from build123d import *

# Parameters (mm, degrees)
SKETCH3_R            = 27.94
BOSS_EXTRUDE2_DEPTH  = 122.46
SKETCH5_R            = 3.175
CUT_EXTRUDE1_DEPTH   = 129.676877488
SKETCH4_W            = 14
SKETCH4_H            = 6
SHELL1_START         = 3
SHELL1_OUTLINE_R     = 10.94
SHELL1_OUTLINE_R_2   = 6.175
SHELL1_DEPTH         = 116.46
SHELL1_2_OUTLINE_R   = 24.94
SHELL1_2_OUTLINE_R_2 = 10.94
SHELL1_2_DEPTH       = 10.72
SHELL1_START_2       = 109.72
SHELL1_3_OUTLINE_R   = 24.94
SHELL1_3_OUTLINE_R_2 = 10.94
SHELL1_3_DEPTH       = 9.74
SHELL1_START_3       = 25.72
SHELL1_4_OUTLINE_R   = 24.94
SHELL1_4_OUTLINE_R_2 = 10.94
SHELL1_4_DEPTH       = 9
SHELL1_START_4       = 46.72
SHELL1_5_OUTLINE_R   = 24.94
SHELL1_5_OUTLINE_R_2 = 10.94
SHELL1_5_DEPTH       = 9
SHELL1_START_5       = 67.72
SHELL1_6_OUTLINE_R   = 24.94
SHELL1_6_OUTLINE_R_2 = 10.94
SHELL1_6_DEPTH       = 9
SHELL1_START_6       = 88.72
SHELL1_7_OUTLINE_R   = 24.94
SHELL1_7_OUTLINE_R_2 = 10.94
SHELL1_7_DEPTH       = 9
BOSS_EXTRUDE3_REACH  = 130.677
SKETCH13_W           = 16.483162312
SKETCH13_H           = 6
CUT_EXTRUDE3_DEPTH   = 123
BOSS_EXTRUDE5_START  = -122.46
BOSS_EXTRUDE5_DEPTH  = 122.46


# Read off the part's stored shape, not the designer's step: Shell1
with BuildPart() as part:
    # Sketch3 → Boss-Extrude2 (new body)
    with BuildSketch(Plane.XY):
        Circle(SKETCH3_R)
    extrude(amount=BOSS_EXTRUDE2_DEPTH)

    # Sketch5 → Cut-Extrude1 (cut, through all)
    with BuildSketch(Plane.XY.offset(122.46)):
        Circle(SKETCH5_R)
    extrude(amount=-CUT_EXTRUDE1_DEPTH, mode=Mode.SUBTRACT)

    # Sketch4 → Cut-Revolve1 (revolve, cut)
    with BuildSketch(Plane(origin=(0, 0, 0), x_dir=(1, 0, 0), z_dir=(0, 1, 0)), mode=Mode.PRIVATE) as cut_revolve1_sk:
        with Locations((-20.94, -103.72)):
            Rectangle(SKETCH4_W, SKETCH4_H)
        with Locations((-20.94, -82.72)):
            Rectangle(SKETCH4_W, SKETCH4_H)
        with Locations((-20.94, -61.72)):
            Rectangle(SKETCH4_W, SKETCH4_H)
        with Locations((-20.94, -40.72)):
            Rectangle(SKETCH4_W, SKETCH4_H)
        with Locations((-20.94, -19.72)):
            Rectangle(SKETCH4_W, SKETCH4_H)
    revolve(cut_revolve1_sk.sketch.rotate(Axis((0, 0, 122.46), (0, 0, -1)), 180), axis=Axis((0, 0, 122.46), (0, 0, -1)), mode=Mode.SUBTRACT)

    # Shell1 outline → Shell1 (cut)
    with BuildSketch(Plane.XY.offset(SHELL1_START)):
        Circle(SHELL1_OUTLINE_R)
        Circle(SHELL1_OUTLINE_R_2, mode=Mode.SUBTRACT)
    extrude(amount=SHELL1_DEPTH, mode=Mode.SUBTRACT)

    # Shell1 2 outline → Shell1 2 (cut)
    with BuildSketch(Plane.XY.offset(SHELL1_START)):
        Circle(SHELL1_2_OUTLINE_R)
        Circle(SHELL1_2_OUTLINE_R_2, mode=Mode.SUBTRACT)
    extrude(amount=SHELL1_2_DEPTH, mode=Mode.SUBTRACT)

    # Shell1 3 outline → Shell1 3 (cut)
    with BuildSketch(Plane.XY.offset(SHELL1_START_2)):
        Circle(SHELL1_3_OUTLINE_R)
        Circle(SHELL1_3_OUTLINE_R_2, mode=Mode.SUBTRACT)
    extrude(amount=SHELL1_3_DEPTH, mode=Mode.SUBTRACT)

    # Shell1 4 outline → Shell1 4 (cut)
    with BuildSketch(Plane.XY.offset(SHELL1_START_3)):
        Circle(SHELL1_4_OUTLINE_R)
        Circle(SHELL1_4_OUTLINE_R_2, mode=Mode.SUBTRACT)
    extrude(amount=SHELL1_4_DEPTH, mode=Mode.SUBTRACT)

    # Shell1 5 outline → Shell1 5 (cut)
    with BuildSketch(Plane.XY.offset(SHELL1_START_4)):
        Circle(SHELL1_5_OUTLINE_R)
        Circle(SHELL1_5_OUTLINE_R_2, mode=Mode.SUBTRACT)
    extrude(amount=SHELL1_5_DEPTH, mode=Mode.SUBTRACT)

    # Shell1 6 outline → Shell1 6 (cut)
    with BuildSketch(Plane.XY.offset(SHELL1_START_5)):
        Circle(SHELL1_6_OUTLINE_R)
        Circle(SHELL1_6_OUTLINE_R_2, mode=Mode.SUBTRACT)
    extrude(amount=SHELL1_6_DEPTH, mode=Mode.SUBTRACT)

    # Shell1 7 outline → Shell1 7 (cut)
    with BuildSketch(Plane.XY.offset(SHELL1_START_6)):
        Circle(SHELL1_7_OUTLINE_R)
        Circle(SHELL1_7_OUTLINE_R_2, mode=Mode.SUBTRACT)
    extrude(amount=SHELL1_7_DEPTH, mode=Mode.SUBTRACT)

    # Boss-Extrude3: up to this face of the body (flat: up to its plane)
    boss_extrude3_end = Plane(part.part.faces().sort_by_distance((-27.149737461, 0, 122.46))[0])
    # Sketch10 → Boss-Extrude3 (add, up to the picked face)
    with BuildSketch(Plane(origin=(0, 0, 0), x_dir=(-1, 0, 0), z_dir=(0, 0, -1)), mode=Mode.PRIVATE) as boss_extrude3_sk1:
        with BuildLine():
            Line((-1, 27.922098775), (-1, 3.01340754))
            ThreePointArc((-1, 3.01340754), (0, 3.175), (1, 3.01340754))
            Line((1, 3.01340754), (1, 27.922098775))
            ThreePointArc((1, 27.922098775), (0, 27.94), (-1, 27.922098775))
        make_face()
    boss_extrude3_tool1 = split(extrude(boss_extrude3_sk1.sketch, amount=-BOSS_EXTRUDE3_REACH, mode=Mode.PRIVATE), bisect_by=boss_extrude3_end, keep=Keep.BOTH, mode=Mode.PRIVATE)
    # Sketch10 → Boss-Extrude3 (add, up to the picked face)
    with BuildSketch(Plane(origin=(0, 0, 0), x_dir=(-1, 0, 0), z_dir=(0, 0, -1)), mode=Mode.PRIVATE) as boss_extrude3_sk2:
        with BuildLine():
            Line((3.01340754, 1), (27.922098775, 1))
            ThreePointArc((27.922098775, 1), (27.94, 0), (27.922098775, -1))
            Line((27.922098775, -1), (3.01340754, -1))
            ThreePointArc((3.01340754, -1), (3.175, 0), (3.01340754, 1))
        make_face()
    boss_extrude3_tool2 = split(extrude(boss_extrude3_sk2.sketch, amount=-BOSS_EXTRUDE3_REACH, mode=Mode.PRIVATE), bisect_by=boss_extrude3_end, keep=Keep.BOTH, mode=Mode.PRIVATE)
    # Sketch10 → Boss-Extrude3 (add, up to the picked face)
    with BuildSketch(Plane(origin=(0, 0, 0), x_dir=(-1, 0, 0), z_dir=(0, 0, -1)), mode=Mode.PRIVATE) as boss_extrude3_sk3:
        with BuildLine():
            Line((-1, -3.01340754), (-1, -27.922098775))
            ThreePointArc((-1, -27.922098775), (0, -27.94), (1, -27.922098775))
            Line((1, -27.922098775), (1, -3.01340754))
            ThreePointArc((1, -3.01340754), (0, -3.175), (-1, -3.01340754))
        make_face()
    boss_extrude3_tool3 = split(extrude(boss_extrude3_sk3.sketch, amount=-BOSS_EXTRUDE3_REACH, mode=Mode.PRIVATE), bisect_by=boss_extrude3_end, keep=Keep.BOTH, mode=Mode.PRIVATE)
    # Sketch10 → Boss-Extrude3 (add, up to the picked face)
    with BuildSketch(Plane(origin=(0, 0, 0), x_dir=(-1, 0, 0), z_dir=(0, 0, -1)), mode=Mode.PRIVATE) as boss_extrude3_sk4:
        with BuildLine():
            Line((-27.922098775, -1), (-3.01340754, -1))
            ThreePointArc((-3.01340754, -1), (-3.175, 0), (-3.01340754, 1))
            Line((-3.01340754, 1), (-27.922098775, 1))
            ThreePointArc((-27.922098775, 1), (-27.94, 0), (-27.922098775, -1))
        make_face()
    boss_extrude3_tool4 = split(extrude(boss_extrude3_sk4.sketch, amount=-BOSS_EXTRUDE3_REACH, mode=Mode.PRIVATE), bisect_by=boss_extrude3_end, keep=Keep.BOTH, mode=Mode.PRIVATE)
    add(boss_extrude3_tool1.solids().sort_by(Axis((0, 15.527819, 0), (0, 0, 1)))[0])
    add(boss_extrude3_tool2.solids().sort_by(Axis((-15.527819, 0, 0), (0, 0, 1)))[0])
    add(boss_extrude3_tool3.solids().sort_by(Axis((0, -15.527819, 0), (0, 0, 1)))[0])
    add(boss_extrude3_tool4.solids().sort_by(Axis((15.527819, 0, 0), (0, 0, 1)))[0])

    # Sketch13 → Cut-Revolve2 (revolve, cut)
    with BuildSketch(Plane(origin=(0, 0, 0), x_dir=(1, 0, 0), z_dir=(0, 1, 0)), mode=Mode.PRIVATE) as cut_revolve2_sk:
        with Locations((-22.145666886, -40.72)):
            Rectangle(SKETCH13_W, SKETCH13_H)
        with Locations((-22.145666886, -19.72)):
            Rectangle(SKETCH13_W, SKETCH13_H)
        with Locations((-22.145666886, -61.72)):
            Rectangle(SKETCH13_W, SKETCH13_H)
        with Locations((-22.145666886, -82.72)):
            Rectangle(SKETCH13_W, SKETCH13_H)
        with Locations((-22.145666886, -103.72)):
            Rectangle(SKETCH13_W, SKETCH13_H)
    revolve(cut_revolve2_sk.sketch.rotate(Axis((0, 0, 121.588746248), (0, 0, -1)), 180), axis=Axis((0, 0, 121.588746248), (0, 0, -1)), mode=Mode.SUBTRACT)

    # Sketch16 → Cut-Extrude3 (cut)
    with BuildSketch(Plane(origin=(0, 0, 0), x_dir=(-1, 0, 0), z_dir=(0, 0, -1))):
        with BuildLine():
            Line((-27.923120749, -0.971044624), (-6.098171639, -0.971044624))
            ThreePointArc((-6.098171639, -0.971044624), (-0.014665674, -6.174982584), (6.093490379, -1))
            Line((6.093490379, -1), (27.922098775, -1))
            ThreePointArc((27.922098775, -1), (-0.014486703, -27.939996244), (-27.923120749, -0.971044624))
        make_face()
    extrude(amount=-CUT_EXTRUDE3_DEPTH, mode=Mode.SUBTRACT)

    # Sketch18 → Boss-Extrude5 (add)
    with BuildSketch(Plane(origin=(0, 0, 0), x_dir=(-1, 0, 0), z_dir=(0, 0, -1)).offset(BOSS_EXTRUDE5_START)):
        with BuildLine():
            Line((-3.175, 0), (-13.90408573, 0))
            ThreePointArc((-13.90408573, 0), (0, -13.90408573), (13.90408573, 0))
            Line((13.90408573, 0), (3.175, 0))
            ThreePointArc((3.175, 0), (0, -3.175), (-3.175, 0))
        make_face()
    extrude(amount=BOSS_EXTRUDE5_DEPTH)


solid = part.part
The listing builds one solid part. Answer for the finished solid, in the listing's coordinates (mm). A direction names the side the tool comes from. Coordinates: 2 decimals unless noted, no trailing zeros. Loops run counter-clockwise (first coordinate to the right, second up) from the corner with the lowest first, then second, coordinate; pieces in that order, holes last.
1) A tool of negligible diameter and unlimited length cuts with its end or side. For faces 1 (the face through (0, 16, 64.72)), 2 (the face through (21, -0.971, 93)), 3 (the face through (-9, 1, 60)), from which of +Z, -Z, +X, -X, +Y, -Y can it reach the whole face along a straight path? Write none if from no direction.
2) Find section D-D on y = -7. Write down the section's boundary in (x, z), then the cut area to 3 significant figures.
3) Determine the mould class of faces 4 (the face through (0, 7, 122.46)), 5 (the face through (0.614, 27.933, 93.115)), 6 (the face through (-17.45, 17.82, 93.16)) for opening direction X: pulls with the +X half, pulls with the -X half, needs draft (parallel to the pull), parting line crosses it, or undercut.
4) Find section A-A on z = 69. Give the number of separate pieces and of enclosed holes in the cut face, then the cut area to 3 significant figures.
5) Flat-ended cylindrical pins translate along their axes: pin 1 Ø6 at (y, z) = (17, 26.5) entering from +X; pin 2 Ø11 at (x, z) = (20, 6.5) entering from -Y; pin 3 Ø6 at (x, y) = (6.5, 9.5) entering from -Z; pin 4 Ø1 at (y, z) = (23.5, 54.5) entering from -X. Find the tip coordinate at first contact, or state that the pin passes through.
6) Find the intervals of material crossed by L1, parallel to Z at x = 5.5, y = 7; L2, parallel to X at y = 13, z = 69.5; L3, parallel to X at y = 9, z = 54, in increasing order.
Values:
1. face 1: +Y
1. face 2: +Z, -Z, +X, -Y
1. face 3: none
2. outline: (-12.01, 0) - (12.01, 0) - (12.01, 122.46) - (-12.01, 122.46) - close
2. area: 2,940 mm2
3. face 4: needs draft
3. face 5: parting line crosses it
3. face 6: undercut
4. separate pieces: 1
4. enclosed holes: 3
4. area: 684 mm2
5. pin 1: stops at x = 24.18
5. pin 2: stops at y = -0.97
5. pin 3: stops at z = 0
5. pin 4: stops at x = -15.86
6. L1: z = 0 to 3, 119.46 to 122.46
6. L2: x = -24.73 to -21.28, -1 to 1, 21.28 to 24.73
6. L3: x = -26.45 to -23.26, -1 to 1, 23.26 to 26.45
